```python
from build123d import *

# Parameters (mm, degrees)
F0_W     = 27
F0_H     = 24.8
F1_DEPTH = 18
F2_W     = 21
F2_H     = 21.8
F3_DEPTH = 15
F5_DEPTH = 14
F7_DEPTH = 10
F8_SIZE  = 1.5


with BuildPart() as f1:
    # F0 (on Top) → F1 (new body)
    with BuildSketch(Plane.XY):
        Rectangle(F0_W, F0_H)
    extrude(amount=F1_DEPTH)

    # F2 (on face) → F3 (cut)
    with BuildSketch(Plane.XY.offset(18)):
        with Locations((0, -1.5)):
            Rectangle(F2_W, F2_H)
    extrude(amount=-F3_DEPTH, mode=Mode.SUBTRACT)

    # F4 (on face) → F5 (join)
    with BuildSketch(Plane.XY.offset(18)):
        with BuildLine():
            ThreePointArc((-10.5, -9.02665), (-10.1, -7.7), (-10.5, -6.37335))
            Line((-10.5, -6.37335), (-10.5, -9.02665))
        make_face()
        with BuildLine():
            ThreePointArc((10.5, -6.37335), (10.1, -7.7), (10.5, -9.02665))
            Line((10.5, -9.02665), (10.5, -6.37335))
        make_face()
    extrude(amount=-F5_DEPTH)

    # F6 (on face) → F7 (cut)
    with BuildSketch(Plane.XZ.offset(12.4)):
        with BuildLine():
            ThreePointArc((10, 12.151472), (10.4, 13), (10, 13.848528))
            Line((10, 13.848528), (10, 12.151472))
        make_face()
        with BuildLine():
            Line((-10, 12.151472), (-10, 13.848528))
            ThreePointArc((-10, 13.848528), (-10.4, 13), (-10, 12.151472))
        make_face()
    extrude(amount=-F7_DEPTH, mode=Mode.SUBTRACT)

    # F8
    f8_edges = [f1.edges().sort_by_distance(p)[0] for p in [
        (13.5, 0, 0),
        (13.5, 0, 18),
        (-13.5, 0, 18),
        (-13.5, 0, 0),
        (-13.5, 12.4, 9),
        (0, 12.4, 0),
        (13.5, -12.4, 9),
        (-13.5, -12.4, 9),
        (13.5, 12.4, 9),
    ]]
    chamfer(f8_edges, length=F8_SIZE)


solid = f1.part
```
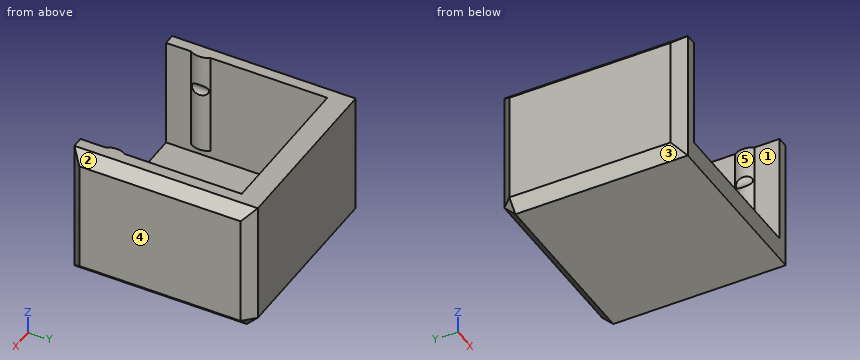
The model under review builds one solid part; all positions refer to its coordinate system, in mm. Face numbers are marked on the shaded views. A direction names the side the tool comes from. Round coordinates to 2 decimals unless told otherwise and drop trailing zeros. Write each loop counter-clockwise with the first axis right and the second up, starting at its lowest first coordinate (ties: lowest second). Pieces come first, ordered by that corner, then holes. Notation, with made-up numbers: M 5,-24 L 42,-24 A18 ccw 42,-9 Z; hole C -11.75,25.25 d1. An arc over 180 degrees is marked long. Use CSV: the item, a comma, the result in double quotes. Start each with the question number.
(1) We need section D-D, the plane z = 13. State the section outline as (x, y) points.
(2) Clearance check with a flat-ended pin moving along its axis: P1, Ø4.5, axis at x = 0.5, z = 10.5, coming from the -Y side. State where the tip first meets the part, or that it passes through.
(3) We need section A-A, the plane y = 2.5. State the section outline as (x, z) points, then the cut area to 4 significant figures.
(4) We need section B-B, the plane z = 9.25. State the section outline as (x, y) points.
(5) For line 1 along X through (y, z) = (6.25, 3.5); line 2 along Z through (x, y) = (-2.5, 8.25); line 3 along Y through (x, z) = (-7.25, 5.5), list the stretches that pass through material, from the lowest coordinate up.
(6) The part is to be moulded in two halves that separate along X. For the marked faces 1, 2 and 3, say which applies: +X half, -X half, draft (parallel to the pull), parting line (faces both ways), or undercut.
(7) Tool access review of the marked faces 4 and 5: name each direction out of +Z, -Z, +X, -X, +Y, -Y from which nothing blocks a thin tool from reaching the whole face with its end or side.
(8) We need section C-C, the plane x = -0.25. State the section outline as (y, z) points.
Findings:
1,outline,"M -13.5,-10.9 L -12,-12.4 L -10.5,-12.4 L -10.5,-9.03 A2.4 ccw -10.4,-8.86 L -10.4,-6.54 A2.4 ccw -10.5,-6.37 L -10.5,9.4 L 10.5,9.4 L 10.5,-6.37 A2.4 ccw 10.4,-6.54 L 10.4,-8.86 A2.4 ccw 10.5,-9.03 L 10.5,-12.4 L 12,-12.4 L 13.5,-10.9 L 13.5,10.9 L 12,12.4 L -12,12.4 L -13.5,10.9 Z"
2,P1,"y = 9.4"
3,outline,"M -13.5,1.5 L -12,0 L 12,0 L 13.5,1.5 L 13.5,16.5 L 12,18 L 10.5,18 L 10.5,3 L -10.5,3 L -10.5,18 L -12,18 L -13.5,16.5 Z"
3,area,"166.5 mm^2"
4,outline,"M -13.5,-10.9 L -12,-12.4 L -10.5,-12.4 L -10.5,-9.03 A2.4 ccw -10.5,-6.37 L -10.5,9.4 L 10.5,9.4 L 10.5,-6.37 A2.4 ccw 10.5,-9.03 L 10.5,-12.4 L 12,-12.4 L 13.5,-10.9 L 13.5,10.9 L 12,12.4 L -12,12.4 L -13.5,10.9 Z"
5,line 1,"-13.5 to -10.5, 10.5 to 13.5"
5,line 2,"0 to 3"
5,line 3,"9.4 to 12.4"
6,face 1,"undercut"
6,face 2,"+X half"
6,face 3,"-X half"
7,face 4,"+Z, -Z, +X, +Y, -Y"
7,face 5,"+Z"
8,outline,"M -12.4,0 L 10.9,0 L 12.4,1.5 L 12.4,18 L 9.4,18 L 9.4,3 L -12.4,3 Z"
